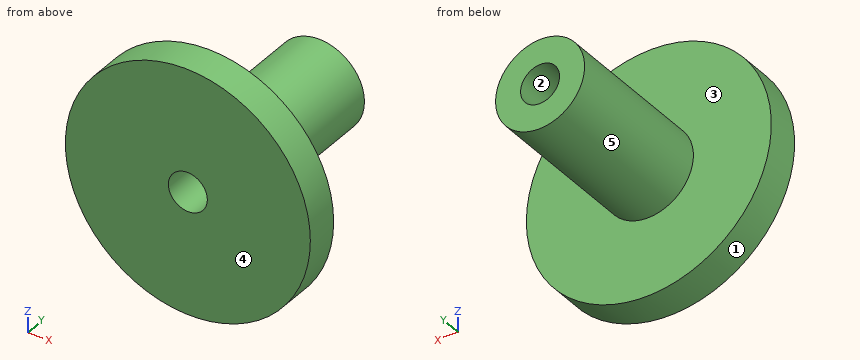
```python
from build123d import *

# Parameters (mm, degrees)
SKETCH1_R           = 11
BOSS_EXTRUDE1_DEPTH = 3
SKETCH2_R           = 4
BOSS_EXTRUDE2_DEPTH = 14
SKETCH3_R           = 1.75
CUT_EXTRUDE1_DEPTH  = 20


with BuildPart() as part:
    # Sketch1 → Boss-Extrude1 (new body)
    with BuildSketch(Plane(origin=(0, 0, 0), x_dir=(1, 0, 0), z_dir=(0, 1, 0))):
        Circle(SKETCH1_R)
    extrude(amount=BOSS_EXTRUDE1_DEPTH)

    # Sketch2 → Boss-Extrude2 (add)
    with BuildSketch(Plane(origin=(0, 3, 0), x_dir=(1, 0, 0), z_dir=(0, 1, 0))):
        Circle(SKETCH2_R)
    extrude(amount=BOSS_EXTRUDE2_DEPTH)

    # Sketch3 → Cut-Extrude1 (cut)
    with BuildSketch(Plane(origin=(0, 17, 0), x_dir=(1, 0, 0), z_dir=(0, 1, 0))):
        Circle(SKETCH3_R)
    extrude(amount=-CUT_EXTRUDE1_DEPTH, mode=Mode.SUBTRACT)


solid = part.part
```
CAD build for the part. Positions are in the model's coordinates, mm. Face numbers are marked on the shaded views. A direction names the side the tool comes from. Round coordinates to 2 decimals unless told otherwise and drop trailing zeros. Write each loop counter-clockwise with the first axis right and the second up, starting at its lowest first coordinate (ties: lowest second). Pieces come first, ordered by that corner, then holes. Notation, with made-up numbers: (82, 79) - (89, 79) arc R13 ccw to (89, 91) - close; hole circle Ø7 at (42.5, 89.5). An arc over 180 degrees is marked (long way). Return JSON: item names as keys, results as strings. Group by question number.
Item 1: 3-axis set-ups, long thin cutter, end or side, ignore diameter. For the marked faces 4 and 5: which of +Z, -Z, +X, -X, +Y, -Y reach the whole face in a straight line?
Item 2: Mould opens along X. For the marked faces 1, 2 and 3 say: +X half, -X half, draft (parallel to the pull), parting line (faces both ways), or undercut.
Item 3: Band-saw the part on B-B on z = 0. List the corners of the cut face in (x, y), plus the area to 4 significant figures.
Item 4: Band-saw the part on D-D on x = -3. List the corners of the cut face in (y, z).
Item 5: Band-saw the part on C-C on y = 1. List the corners of the cut face in (x, z), plus the area to 3 significant figures.
Item 6: Flat gauge pins, fed straight in: pin 1 Ø2 at (y, z) = (4.5, 6) entering from +X; pin 2 Ø3 at (y, z) = (6, 3) entering from -X; pin 3 Ø5 at (y, z) = (15, 3) entering from +X; pin 4 Ø1.5 at (y, z) = (3, -5) entering from -X. Where does each tip first touch, or does it go through?
Item 7: Probe probe 1 along Z at (x, y) = (0, 7); probe 2 along Y at (x, z) = (-7, 4). List the from-to ranges inside material, lowest first.
Item 8: Band-saw the part on A-A on x = 0. List the corners of the cut face in (y, z).
Resolved:
{
 "1": {"face 4": "+Z, -Z, +X, -X, -Y", "face 5": "+Y"},
 "2": {"face 1": "parting line", "face 2": "undercut", "face 3": "draft"},
 "3": {"outline": "(-11, 0) - (-1.75, 0) - (-1.75, 17) - (-4, 17) - (-4, 3) - (-11, 3) - close; (1.75, 0) - (11, 0) - (11, 3) - (4, 3) - (4, 17) - (1.75, 17) - close", "area": "118.5 mm²"},
 "4": {"outline": "(0, -10.58) - (3, -10.58) - (3, -2.65) - (17, -2.65) - (17, 2.65) - (3, 2.65) - (3, 10.58) - (0, 10.58) - close"},
 "5": {"outline": "circle Ø22 at (0, 0); hole circle Ø3.5 at (0, 0)", "area": "371 mm²"},
 "6": {"pin 1": "passes through", "pin 2": "stops at x = -3.71", "pin 3": "stops at x = 3.97", "pin 4": "stops at x = -10.15"},
 "7": {"probe 1": "z = -4 to -1.75, 1.75 to 4", "probe 2": "y = 0 to 3"},
 "8": {"outline": "(0, -11) - (3, -11) - (3, -4) - (17, -4) - (17, -1.75) - (0, -1.75) - close; (0, 1.75) - (17, 1.75) - (17, 4) - (3, 4) - (3, 11) - (0, 11) - close"}
}
